For this review, use the dimensioned drawing (mm, ordinates from the lowest corner) and the shaded views. Coordinates: 2 decimals unless noted, no trailing zeros. Order: outer loops, then holes, each group sorted by start corner. A loop starts at its lowest first (then second) coordinate and runs counter-clockwise, first axis right, second up. Notation, with made-up numbers: (-19.5, 44) -> (7.5, 44) arc R20 cw to (7.5, 66) -> close; hole circle Ø6 at (42.5, -22). An arc over 180 degrees is marked (long way). Return JSON: item names as keys, results as strings. Group by question number.
Item 1: For line 1 along Y through (x, z) = (25, 8.75); line 2 along Y through (x, z) = (25, 11.75); line 3 along Z through (x, y) = (26.5, 11.25), list the stretches that pass through material, from the lowest coordinate up.
Item 2: Take a section at C-C (z = 13.25). Write out the cut boundary in (x, y), then the cut area to 3 significant figures.
Item 3: Take a section at A-A (x = 25). Write out the cut boundary in (y, z), then the cut area to 3 significant figures.
Item 4: Take a section at D-D (x = 39.5). Write out the cut boundary in (y, z), then the cut area to 3 significant figures.
Item 5: Take a section at B-B (y = 12.5). Write out the cut boundary in (x, z), then the cut area to 3 significant figures.
Item 6: Insertion check: pin 1 (3 mm diameter, centred on x = 6, y = 11, fed in from +Z). The pin has a flat end and moves straight along its axis. Give the tip position at first contact, or say it passes through.
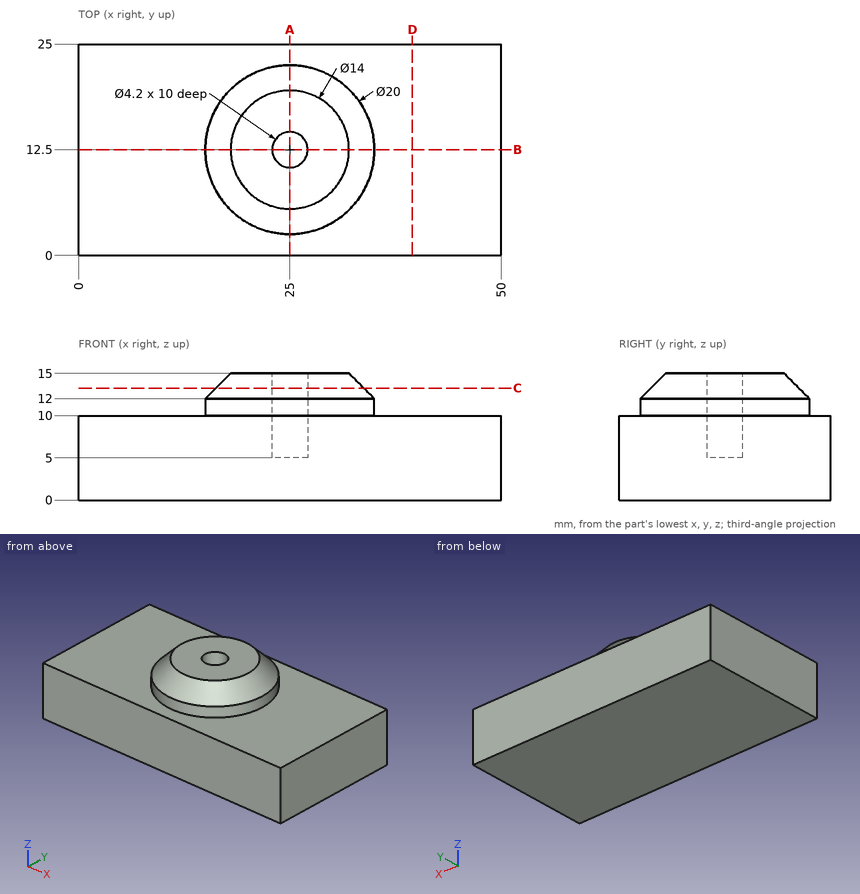
Findings below:
{
 "1": {"line 1": "y = 0 to 10.4, 14.6 to 25", "line 2": "y = 2.5 to 10.4, 14.6 to 22.5", "line 3": "z = 0 to 5"},
 "2": {"outline": "circle Ø17.5 at (25, 12.5); hole circle Ø4.2 at (25, 12.5)", "area": "227 mm2"},
 "3": {"outline": "(0, 0) -> (25, 0) -> (25, 10) -> (22.5, 10) -> (22.5, 12) -> (19.5, 15) -> (14.6, 15) -> (14.6, 5) -> (10.4, 5) -> (10.4, 15) -> (5.5, 15) -> (2.5, 12) -> (2.5, 10) -> (0, 10) -> close", "area": "299 mm2"},
 "4": {"outline": "(0, 0) -> (25, 0) -> (25, 10) -> (0, 10) -> close", "area": "250 mm2"},
 "5": {"outline": "(0, 0) -> (50, 0) -> (50, 10) -> (35, 10) -> (35, 12) -> (32, 15) -> (27.1, 15) -> (27.1, 5) -> (22.9, 5) -> (22.9, 15) -> (18, 15) -> (15, 12) -> (15, 10) -> (0, 10) -> close", "area": "549 mm2"},
 "6": {"pin 1": "stops at z = 10"}
}
